Part model, mm, in its own coordinate system. Coordinates: 2 decimals unless noted, no trailing zeros. Order: outer loops, then holes, each group sorted by start corner. A loop starts at its lowest first (then second) coordinate and runs counter-clockwise, first axis right, second up. Notation, with made-up numbers: M -35.75,15.5 L 20.25,15.5 A28 ccw 20.25,33.5 Z; hole C 55.25,-14 d7. An arc over 180 degrees is marked long. Write item = value, one per line. Start each with the question number.
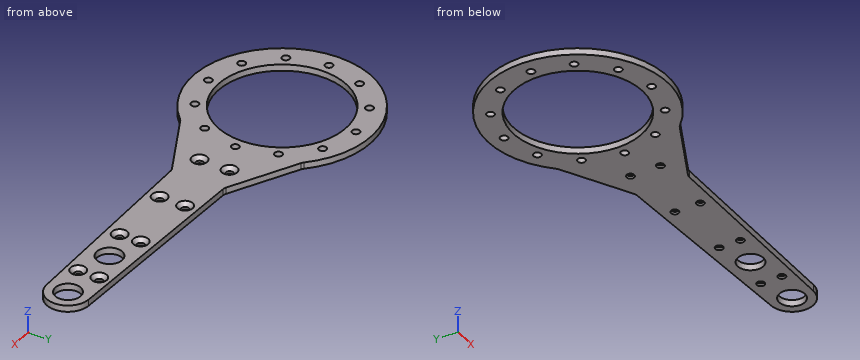
from build123d import *

# Parameters (mm, degrees)
SKETCH1_R               = 15.1
SKETCH1_R_2             = 3
BOSS_EXTRUDE1_DEPTH     = 1.5
D_GAGEMENT_M1_62_D      = 1.8
D_GAGEMENT_M1_62_DEPTH  = 11.5
CIRPATTERN1_COUNT       = 12
CHAMFER2_SIZE           = 11.480741847
FILLET4_R               = 2
D_GAGEMENT_M1_61_D      = 1.8
D_GAGEMENT_M1_61_DEPTH  = 11.5
CHAMFER3_SIZE           = 0.9
ESQUISSE1_R             = 0.9
ENL_V_MAT_EXTRU_1_DEPTH = 10
CHANFREIN1_SIZE         = 0.9
ESQUISSE2_R             = 0.9
ENL_V_MAT_EXTRU_2_DEPTH = 10
CHANFREIN2_SIZE         = 0.9


with BuildPart() as part:
    # Sketch1 → Boss-Extrude1 (new body)
    with BuildSketch(Plane.XY):
        with BuildLine():
            Line((19.968725548, 6.5), (80.124766302, 4.998443095))
            ThreePointArc((80.124766302, 4.998443095), (85, 0), (80.124766302, -4.998443095))
            Line((80.124766302, -4.998443095), (19.968725548, -6.5))
            ThreePointArc((19.968725548, -6.5), (-21, 0), (19.968725548, 6.5))
        make_face()
        Circle(SKETCH1_R, mode=Mode.SUBTRACT)
        with Locations((64.5, 0)):
            Circle(SKETCH1_R_2, mode=Mode.SUBTRACT)
        with Locations((80, 0)):
            Circle(SKETCH1_R_2, mode=Mode.SUBTRACT)
    extrude(amount=BOSS_EXTRUDE1_DEPTH)

    # Dégagement M1.62
    with Locations(Plane.XY.offset(1.5)):
        with Locations((0, 17.5)):
            d_gagement_m1_62 = Hole(D_GAGEMENT_M1_62_D / 2, depth=D_GAGEMENT_M1_62_DEPTH)

    # CirPattern1: Dégagement M1.62 ×12 about axis
    cirpattern1_axis = Axis((0, 0, 0), (0, 0, 1))
    for i in range(1, CIRPATTERN1_COUNT):
        add(d_gagement_m1_62.rotate(cirpattern1_axis, i * 360 / CIRPATTERN1_COUNT), mode=Mode.SUBTRACT)

    # Chamfer2
    # the kernel refuses this chamfer: 11.480741847, 7 mm, written as the material it adds along each edge
    with BuildSketch(Plane(origin=(19.968725548, -6.5, 0), x_dir=(-0.5119667812352321, -0.8590052473132141, 0), z_dir=(0, 0, 1))) as chamfer2_piece_1:
        with BuildLine():
            Line((9.279580073, 0), (-CHAMFER2_SIZE * 0.533242346076, CHAMFER2_SIZE * 0.845962528924))
            Line((-CHAMFER2_SIZE * 0.533242346076, CHAMFER2_SIZE * 0.845962528924), (0, 0))
            ThreePointArc((0, 0), (4.840122862, 0.518020319), (9.279580073, 0))
        make_face()
    extrude(amount=1.5)
    with BuildSketch(Plane(origin=(19.968725548, 6.5, 0), x_dir=(0.9996886189188567, -0.024953260390352783, 0), z_dir=(0, 0, 1))) as chamfer2_piece_2:
        with BuildLine():
            Line((CHAMFER2_SIZE, 0), (-4.948265049, 7.850177026))
            ThreePointArc((-4.948265049, 7.850177026), (-2.142732691, 4.370792947), (0, 0))
            Line((0, 0), (CHAMFER2_SIZE, 0))
        make_face()
    extrude(amount=1.5)

    # Fillet4
    fillet4_edges = [part.edges().sort_by_distance(p)[0] for p in [
        (31.445892509, -6.213518059, 0.75),
        (15.217888807, 14.471207976, 0.75),
        (15.217888807, -14.471207976, 0.75),
        (31.445892509, 6.213518059, 0.75),
    ]]
    fillet(fillet4_edges, radius=FILLET4_R)

    # Dégagement M1.61
    with Locations(Plane.XY.offset(1.5)):
        with Locations((56.75, 2.5), (72.25, 2.5), (72.25, -2.5), (56.75, -2.5)):
            Hole(D_GAGEMENT_M1_61_D / 2, depth=D_GAGEMENT_M1_61_DEPTH)

    # Chamfer3
    chamfer3_edges = [part.edges().sort_by_distance(p)[0] for p in [
        (57.65, -2.5, 1.5),
        (73.15, -2.5, 1.5),
        (73.15, 2.5, 1.5),
        (57.65, 2.5, 1.5),
    ]]
    chamfer(chamfer3_edges, length=CHAMFER3_SIZE)

    # Esquisse1 → Enlèv. mat.-Extru.1 (cut)
    with BuildSketch(Plane.XY.offset(1.5)):
        with Locations((25.251835753, 3.548914074)):
            Circle(ESQUISSE1_R)
        with Locations((25.251835753, -3.548914074)):
            Circle(ESQUISSE1_R)
    extrude(amount=-ENL_V_MAT_EXTRU_1_DEPTH, mode=Mode.SUBTRACT)

    # Chanfrein1
    chanfrein1_edges = [part.edges().sort_by_distance(p)[0] for p in [
        (24.351835753, 3.548914074, 1.5),
        (24.351835753, -3.548914074, 1.5),
    ]]
    chamfer(chanfrein1_edges, length=CHANFREIN1_SIZE)

    # Esquisse2 → Enlèv. mat.-Extru.2 (cut)
    with BuildSketch(Plane.XY.offset(1.5)):
        with Locations((41.000917876, 3.024457037)):
            Circle(ESQUISSE2_R)
        with Locations((41.000917876, -3.024457037)):
            Circle(ESQUISSE2_R)
    extrude(amount=-ENL_V_MAT_EXTRU_2_DEPTH, mode=Mode.SUBTRACT)

    # Chanfrein2
    chanfrein2_edges = [part.edges().sort_by_distance(p)[0] for p in [
        (40.100917876, 3.024457037, 1.5),
        (40.100917876, -3.024457037, 1.5),
    ]]
    chamfer(chanfrein2_edges, length=CHANFREIN2_SIZE)


solid = part.part
Item 1: Cut at C-C, the plane x = 69. Write the cut outline in (y, z), and give its area (3 significant figures).
Item 2: Cut at B-B, the plane x = -5.5. Write the cut outline in (y, z), and give its area (3 significant figures).
Item 3: Wall check: line 1 along Y through (x, z) = (0, 0.3); line 2 along X through (y, z) = (-13, 0.45); line 3 along Y through (x, z) = (-12, 0.9). Give the ranges that are in metal, low to high. Write a range as [from, to].
Item 4: Flat gauge pins, fed straight in: pin 1 (2 mm diameter, centred on x = 41, y = -3.02, fed in from +Z); pin 2 (3 mm diameter, centred on x = 56.75, y = 2.5, fed in from +Z); pin 3 (2.5 mm diameter, centred on x = 41, y = 3.02, fed in from +Z). Where does each tip first touch, or does it go through?
Item 5: Cut at A-A, the plane z = 0.3. Count the separate pieces of the cut face and the enclosed holes in it, and give its area (3 significant figures).
Filled sheet:
q1.outline = M -5.28,0 L 5.28,0 L 5.28,1.5 L -5.28,1.5 Z
q1.area = 15.8 mm2
q2.outline = M -20.27,0 L -14.06,0 L -14.06,1.5 L -20.27,1.5 Z; M 14.06,0 L 20.27,0 L 20.27,1.5 L 14.06,1.5 Z
q2.area = 18.6 mm2
q3.line_1 = [-21, -18.4], [-16.6, -15.1], [15.1, 16.6], [18.4, 21]
q3.line_2 = [-16.49, -7.68], [7.68, 18.11]
q3.line_3 = [-17.23, -9.17], [9.17, 17.23]
q4.pin_1 = 0.7
q4.pin_2 = 1.2
q4.pin_3 = 0.95
q5.separate_pieces = 1
q5.enclosed_holes = 23
q5.area = 1,370 mm2
